```python
from build123d import *

# Parameters (mm, degrees)
SKETCH1_R           = 14
SKETCH1_R_2         = 1.5
BOSS_EXTRUDE1_DEPTH = 3
SKETCH2_R           = 7.5
BOSS_EXTRUDE2_DEPTH = 13
FILLET1_R           = 1
CUT_EXTRUDE2_START  = -6
SKETCH4_R           = 2.6
CUT_EXTRUDE2_DEPTH  = 6


with BuildPart() as part:
    # Sketch1 → Boss-Extrude1 (new body)
    with BuildSketch(Plane(origin=(0, 0, 0), x_dir=(1, 0, 0), z_dir=(0, 1, 0))):
        with Locations(Location((0, 0, 0), (0, 0, 270))):
            Circle(SKETCH1_R)
        with Locations(Location((0, 10.5, 0), (0, 0, 270))):
            Circle(SKETCH1_R_2, mode=Mode.SUBTRACT)
        with Locations(Location((10.5, 0, 0), (0, 0, 270))):
            Circle(SKETCH1_R_2, mode=Mode.SUBTRACT)
        with Locations(Location((0, -10.5, 0), (0, 0, 270))):
            Circle(SKETCH1_R_2, mode=Mode.SUBTRACT)
        with Locations(Location((-10.5, 0, 0), (0, 0, 270))):
            Circle(SKETCH1_R_2, mode=Mode.SUBTRACT)
        with BuildLine():
            Line((-2.35, 1.112429773), (-2.35, -1.112429773))
            ThreePointArc((-2.35, -1.112429773), (2.6, 0), (-2.35, 1.112429773))
        make_face(mode=Mode.SUBTRACT)
    extrude(amount=BOSS_EXTRUDE1_DEPTH)

    # Sketch2 → Boss-Extrude2 (add)
    with BuildSketch(Plane(origin=(0, 3, 0), x_dir=(1, 0, 0), z_dir=(0, 1, 0))):
        with Locations(Location((0, 0, 0), (0, 0, 90))):
            Circle(SKETCH2_R)
        with BuildLine():
            Line((-2.35, 1.112429773), (-2.35, -1.112429773))
            ThreePointArc((-2.35, -1.112429773), (2.6, 0), (-2.35, 1.112429773))
        make_face(mode=Mode.SUBTRACT)
    extrude(amount=BOSS_EXTRUDE2_DEPTH)

    # Fillet1
    fillet1_edges = [part.edges().sort_by_distance(p)[0] for p in [
        (0, 3, 7.5),
        (0, 16, 7.5),
    ]]
    fillet(fillet1_edges, radius=FILLET1_R)

    # Sketch4 → Cut-Extrude2 (cut)
    with BuildSketch(Plane(origin=(0, 16, 0), x_dir=(1, 0, 0), z_dir=(0, 1, 0)).offset(CUT_EXTRUDE2_START)):
        with Locations(Location((0, 0, 0), (0, 0, 154.668324983))):
            Circle(SKETCH4_R)
    extrude(amount=CUT_EXTRUDE2_DEPTH, mode=Mode.SUBTRACT)


solid = part.part
```
For this review, take the finished solid that the model builds, in its own axes (mm). A direction names the side the tool comes from. Coordinates: 2 decimals unless noted, no trailing zeros. Write each loop counter-clockwise with the first axis right and the second up, starting at its lowest first coordinate (ties: lowest second). Pieces come first, ordered by that corner, then holes.
(1) The part is to be moulded in two halves that separate along Z. For faces 1 (the face through (0, 1, -12)), 2 (the face through (-0.33, 9.423, 7.493)), 3 (the face through (0, 0, 3)), say which applies: +Z half, -Z half, draft (parallel to the pull), parting line (faces both ways), or undercut.
(2) Add section D-D on y = 11.25. Give the boundary of the cut face in (x, z).
(3) For pin 1 Ø6 at (x, z) = (-4, -4) entering from -Y; pin 2 Ø2.5 at (y, z) = (5.5, 0) entering from +X; pin 3 Ø2 at (y, z) = (6.5, -4) entering from +X; pin 4 Ø8 at (x, y) = (-6.5, 12) entering from -Z, all flat-tipped, find the tip position at first contact; note any pin that passes through.
(4) Tool access review of faces 4 (the face through (-6, 3, -6.4)), 5 (the face through (-2.35, 5, 0)), 6 (the face through (0, 16, -3)): name each direction out of +Z, -Z, +X, -X, +Y, -Y from which nothing blocks a thin tool from reaching the whole face with its end or side.
(5) Add section A-A on x = 0. Give the boundary of the cut face in (y, z).
(6) Wall thickness on probe 1 along X at (y, z) = (1.45, 0); probe 2 along Y at (x, z) = (-6.75, 10.5); probe 3 along X at (y, z) = (12, -1): over which ranges is each line inside the solid? List them lowest first.
(7) Add section B-B on z = 0. Give the boundary of the cut face in (x, y).
(8) Add section C-C on y = 2.5. Give the boundary of the cut face in (x, z), then the cut area to 3 significant figures.
Answer sheet:
1. face 1: undercut
1. face 2: parting line
1. face 3: draft
2. outline: circle Ø15 at (0, 0); hole circle Ø5.2 at (0, 0)
3. pin 1: stops at y = 0
3. pin 2: stops at x = 7.5
3. pin 3: stops at x = 6.87
3. pin 4: stops at z = -7.07
4. face 4: +Y
4. face 5: +Y, -Y
4. face 6: +Z, -Z, +X, -X, +Y
5. outline: (0, -14) - (3, -14) - (3, -12) - (0, -12) - close; (0, -9) - (3, -9) - (3, -8.5) arc R1 cw to (4, -7.5) - (15, -7.5) arc R1 ccw to (16, -6.5) - (16, -2.6) - (0, -2.6) - close; (0, 2.6) - (16, 2.6) - (16, 6.5) arc R1 ccw to (15, 7.5) - (4, 7.5) arc R1 cw to (3, 8.5) - (3, 9) - (0, 9) - close; (0, 12) - (3, 12) - (3, 14) - (0, 14) - close
6. probe 1: x = -14 to -12, -9 to -2.35, 2.6 to 9, 12 to 14
6. probe 2: y = 0 to 3
6. probe 3: x = -7.43 to -2.4, 2.4 to 7.43
7. outline: (-14, 0) - (-12, 0) - (-12, 3) - (-14, 3) - close; (-9, 0) - (-2.35, 0) - (-2.35, 10) - (-2.6, 10) - (-2.6, 16) - (-6.5, 16) arc R1 ccw to (-7.5, 15) - (-7.5, 4) arc R1 cw to (-8.5, 3) - (-9, 3) - close; (2.6, 0) - (9, 0) - (9, 3) - (8.5, 3) arc R1 cw to (7.5, 4) - (7.5, 15) arc R1 ccw to (6.5, 16) - (2.6, 16) - close; (12, 0) - (14, 0) - (14, 3) - (12, 3) - close
8. outline: circle Ø28 at (0, 0); hole circle Ø3 at (-10.5, 0); hole (-2.35, -1.11) arc R2.6 ccw (long way) to (-2.35, 1.11) - close; hole circle Ø3 at (0, -10.5); hole circle Ø3 at (0, 10.5); hole circle Ø3 at (10.5, 0)
8. area: 567 mm2
